Job drawing, mm, ordinate dimensions from the low corner. One solid piece. A direction names the side the tool comes from. Give positions to 0.01 mm unless a question says otherwise; leave off trailing zeros. Order: outer loops, then holes, each group sorted by start corner. A loop starts at its lowest first (then second) coordinate and runs counter-clockwise, first axis right, second up. Notation, with made-up numbers: M -4.5,31 L 15.5,31 A13 ccw 15.5,42 Z; hole C 0,10.5 d6. An arc over 180 degrees is marked long. Put each result on its own line as item: value. Start each with the question number.
1) Cut at B-B (z = 8). Write the cut outline in (x, y), and give its area (3 significant figures).
2) Cut at C-C (y = 73). Write the cut outline in (x, z), and give its area (3 significant figures).
3) Cut at A-A (x = 70). Write the cut outline in (y, z), and give its area (3 significant figures).
4) Two-plate mould, pull along Y, no slides. Class the marked faces 1, 2 and 3: released by +Y, released by -Y, zero draft, split by the parting line, or undercut.
5) Pin check, flat tips, straight feed: pin 1 (1.5 mm diameter, centred on y = 29.5, z = 5, fed in from +X); pin 2 (1 mm diameter, centred on x = 21.5, z = 7.5, fed in from -Y); pin 3 (5 mm diameter, centred on y = 66, z = 4, fed in from -X). Stop position of each tip, or through.
6) Drill centre lines: line 1 (Y direction, x = 72, z = 6.75); line 2 (X direction, y = 61.5, z = 7.5); line 3 (Y direction, x = 59.5, z = 4.75). Where is each one in solid material? Low to high. Write a range as [from, to].
7) Tool access for the marked faces 4, 5 and 6: list every direction of +Z, -Z, +X, -X, +Y, -Y with a clear straight run to the whole face (end or side of a thin tool).
8) Cut at D-D (x = 55.5). Write the cut outline in (y, z).
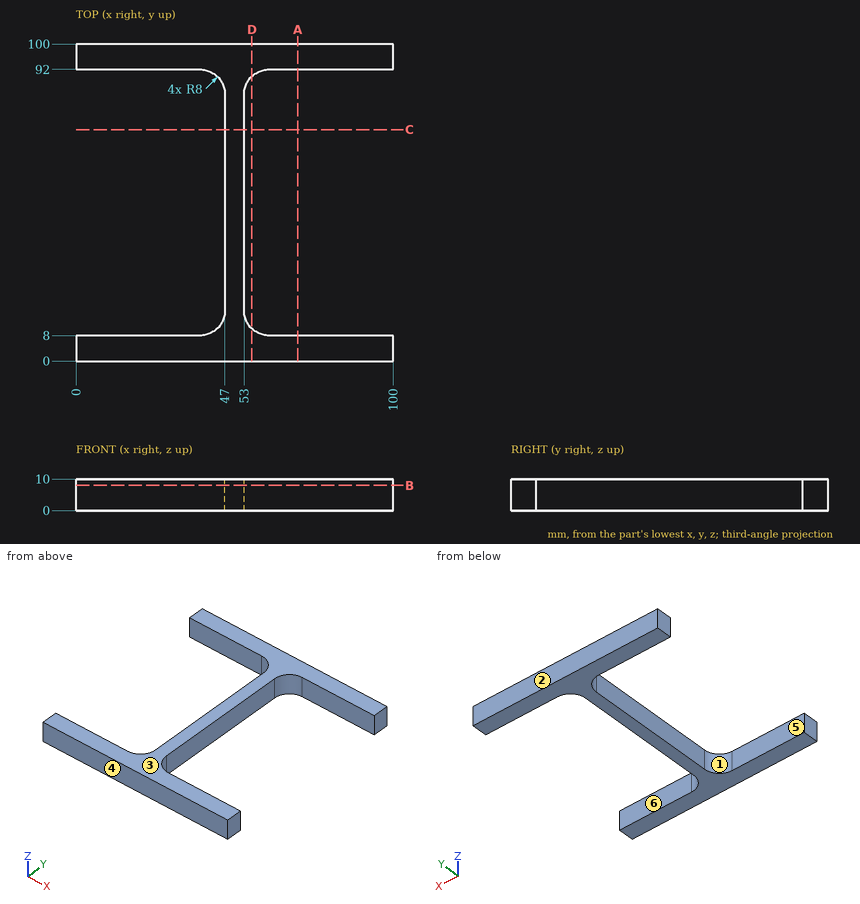
Solution:
1. outline: M 0,0 L 100,0 L 100,8 L 61,8 A8 cw 53,16 L 53,84 A8 cw 61,92 L 100,92 L 100,100 L 0,100 L 0,92 L 39,92 A8 cw 47,84 L 47,16 A8 cw 39,8 L 0,8 Z
1. area: 2,160 mm²
2. outline: M 47,0 L 53,0 L 53,10 L 47,10 Z
2. area: 60.0 mm²
3. outline: M 0,0 L 8,0 L 8,10 L 0,10 Z; M 92,0 L 100,0 L 100,10 L 92,10 Z
3. area: 160 mm²
4. face 1: undercut
4. face 2: released by +Y
4. face 3: zero draft
5. pin 1: x = 53
5. pin 2: y = 0
5. pin 3: x = 47
6. line 1: [0, 8], [92, 100]
6. line 2: [47, 53]
6. line 3: [0, 8.14], [91.86, 100]
7. face 4: +Z, -Z, +X, -X, -Y
7. face 5: +Z, -Z, -X
7. face 6: +Z, -Z, +X
8. outline: M 0,0 L 10.19,0 L 10.19,10 L 0,10 Z; M 89.81,0 L 100,0 L 100,10 L 89.81,10 Z
